Job drawing, mm, ordinate dimensions from the low corner. One solid piece. Round coordinates to 2 decimals unless told otherwise and drop trailing zeros. Write each loop counter-clockwise with the first axis right and the second up, starting at its lowest first coordinate (ties: lowest second). Pieces come first, ordered by that corner, then holes. Notation, with made-up numbers: M 39,-31 L 84,-31 A15 ccw 84,-2 Z; hole C 76,-39.5 d7. An arc over 180 degrees is marked long. Answer as a JSON object with one key per item and string values. Group by question number.
1. Drill centre lines: line 1 (Y direction, x = 15.75, z = 27); line 2 (Y direction, x = 18.25, z = 20); line 3 (Z direction, x = 10.25, y = 76.2). Where is each one in solid material? Low to high. Write a range as from..to.
2. Band-saw the part on C-C, the plane z = 5.5. Write the cut outline in (x, y), plus the area to 3 significant figures.
3. Band-saw the part on B-B, the plane x = 20. Write the cut outline in (y, z).
4. Band-saw the part on A-A, the plane y = 76.2. Write the cut outline in (x, z), plus the area to 3 significant figures.
5. Drop a flat-ended pin along its axis: pin 1 (4 mm diameter, centred on x = 7.5, z = 36.5, fed in from +Y). Give the stop position or say it passes through.
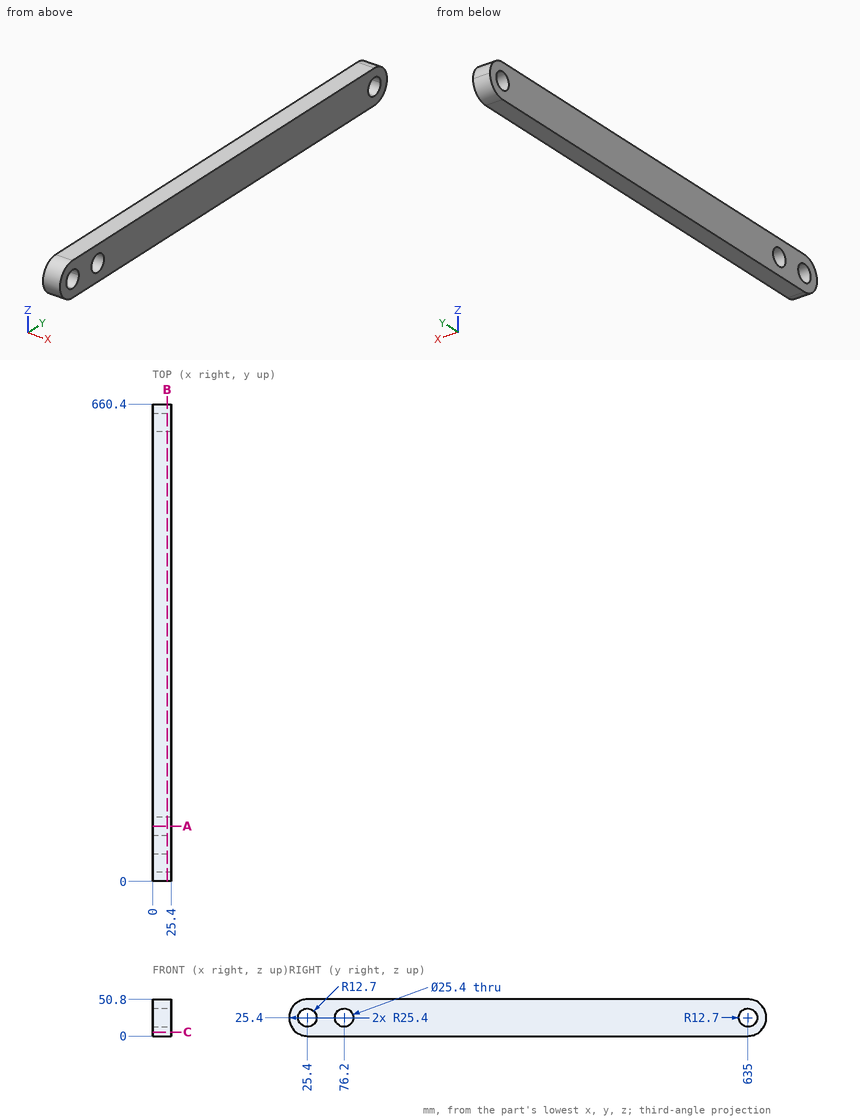
Worked answers:
{
 "1": {"line 1": "y = 0.05..12.8, 38..63.6, 88.8..622.4, 647.6..660.35", "line 2": "y = 0.58..13.91, 36.89..64.71, 87.69..623.51, 646.49..659.82", "line 3": "z = 0..12.7, 38.1..50.8"},
 "2": {"outline": "M 0,9.62 L 25.4,9.62 L 25.4,650.78 L 0,650.78 Z", "area": "16,300 mm^2"},
 "3": {"outline": "M 25.4,0 L 635,0 A25.4 ccw 635,50.8 L 25.4,50.8 A25.4 ccw Z; hole C 25.4,25.4 d25.4; hole C 76.2,25.4 d25.4; hole C 635,25.4 d25.4"},
 "4": {"outline": "M 0,0 L 25.4,0 L 25.4,12.7 L 0,12.7 Z; M 0,38.1 L 25.4,38.1 L 25.4,50.8 L 0,50.8 Z", "area": "645 mm^2"},
 "5": {"pin 1": "stops at y = 658.71"}
}
